Part print with two shaded views. Sizes in mm from the minimum x, y, z corner. A direction names the side the tool comes from. Round coordinates to 2 decimals unless told otherwise and drop trailing zeros. Loops run counter-clockwise (first coordinate to the right, second up) from the corner with the lowest first, then second, coordinate; pieces in that order, holes last. Notation, with made-up numbers: (48.5, 5.5) -> (101.5, 5.5) arc R20 cw to (101.5, 38.5) -> close; hole circle Ø9 at (75, 36.5). An arc over 180 degrees is marked (long way). Use a Markdown table: item, result. Add a question column.
Item 1: Cut at A-A, the plane y = 6.5. List the corners of the cut face in (x, z), plus the area to 3 significant figures.
Item 2: Which spindle directions (+Z, -Z, +X, -X, +Y, -Y) get a long thin tool onto all of the face, cutting with end or side? Do the marked faces 1, 2, 3 and 4. Say none if no direction does.
Item 3: Probe line 1 (X direction, y = 1.25, z = 3.1); line 2 (X direction, y = 3, z = 3.1); line 3 (X direction, y = 5.5, z = 3.5). List the from-to ranges inside material, lowest first. Write a range as [from, to].
Item 4: Flat gauge pins, fed straight in: pin 1 (8.5 mm diameter, centred on x = 25.5, z = 11, fed in from +Y); pin 2 (1 mm diameter, centred on x = 17, z = 7.5, fed in from -Y); pin 3 (2.5 mm diameter, centred on y = 3, z = 4.5, fed in from +X); pin 4 (3.5 mm diameter, centred on x = 35.65, z = 3.1, fed in from +Y). Where does each tip first touch, or does it go through?
Item 5: Cut at D-D, the plane x = 21. List the corners of the cut face in (y, z).
Item 6: Cut at B-B, the plane x = 16.75. List the corners of the cut face in (y, z).
Item 7: Cut at C-C, the plane z = 3.1. List the corners of the cut face in (x, y), plus the area to 3 significant figures.
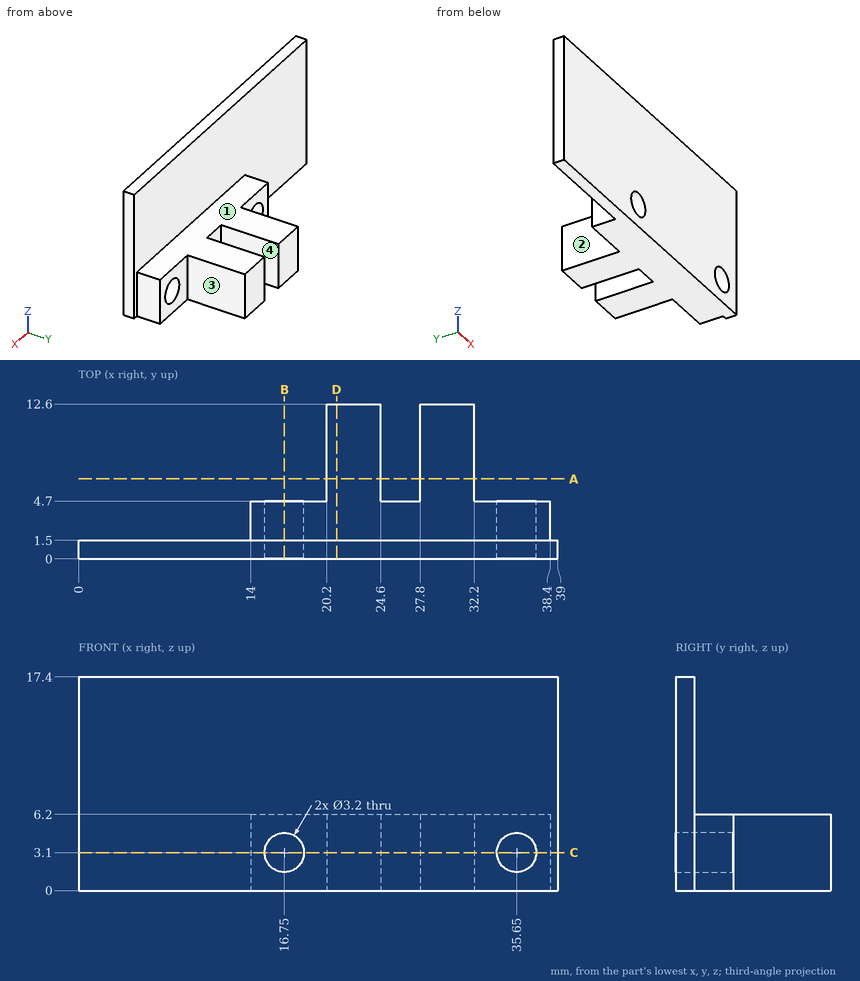
A:
| question | item | result |
|---|---|---|
| 1 | outline | (20.2, 0) -> (24.6, 0) -> (24.6, 6.2) -> (20.2, 6.2) -> close; (27.8, 0) -> (32.2, 0) -> (32.2, 6.2) -> (27.8, 6.2) -> close |
| 1 | area | 54.6 mm^2 |
| 2 | face 1 | +Z, +X, -X, +Y |
| 2 | face 2 | +Z, -Z, -X, +Y |
| 2 | face 3 | +Z, -Z, +X, +Y |
| 2 | face 4 | +Z, -Z, +Y |
| 3 | line 1 | x = [0, 15.15], [18.35, 34.05], [37.25, 39] |
| 3 | line 2 | x = [14, 15.15], [18.35, 34.05], [37.25, 38.4] |
| 3 | line 3 | x = [20.2, 24.6], [27.8, 32.2] |
| 4 | pin 1 | stops at y = 1.5 |
| 4 | pin 2 | stops at y = 0 |
| 4 | pin 3 | stops at x = 38.4 |
| 4 | pin 4 | stops at y = 4.7 |
| 5 | outline | (0, 0) -> (12.6, 0) -> (12.6, 6.2) -> (1.5, 6.2) -> (1.5, 17.4) -> (0, 17.4) -> close |
| 6 | outline | (0, 0) -> (4.7, 0) -> (4.7, 1.5) -> (0, 1.5) -> close; (0, 4.7) -> (4.7, 4.7) -> (4.7, 6.2) -> (1.5, 6.2) -> (1.5, 17.4) -> (0, 17.4) -> close |
| 7 | outline | (0, 0) -> (15.15, 0) -> (15.15, 4.7) -> (14, 4.7) -> (14, 1.5) -> (0, 1.5) -> close; (18.35, 0) -> (34.05, 0) -> (34.05, 4.7) -> (32.2, 4.7) -> (32.2, 12.6) -> (27.8, 12.6) -> (27.8, 4.7) -> (24.6, 4.7) -> (24.6, 12.6) -> (20.2, 12.6) -> (20.2, 4.7) -> (18.35, 4.7) -> close; (37.25, 0) -> (39, 0) -> (39, 1.5) -> (38.4, 1.5) -> (38.4, 4.7) -> (37.25, 4.7) -> close |
| 7 | area | 176 mm^2 |
